Work out the finished part from the listing and answer in its coordinate system (mm). A direction names the side the tool comes from. Round coordinates to 2 decimals unless told otherwise and drop trailing zeros. Write each loop counter-clockwise with the first axis right and the second up, starting at its lowest first coordinate (ties: lowest second). Pieces come first, ordered by that corner, then holes.
1. Determine the mould class of faces 1 (the face through (-169.614, 76.799, -15.023)), 2 (the face through (-172, 11, 35.041)), 3 (the face through (-201.796, 35, 16)) for opening direction X: pulls with the +X half, pulls with the -X half, needs draft (parallel to the pull), parting line crosses it, or undercut.
2. Find section D-D (y = 57). Write down the section's boundary in (x, z), and give its area (3 significant figures).
3. Flat-ended cylindrical pins translate along their axes: pin 1 Ø4.5 at (x, z) = (-192.8, 27.04) entering from +Y; pin 2 Ø8 at (x, z) = (-194.5, 28.5) entering from +Y; pin 3 Ø5.5 at (x, z) = (-150.8, 17.04) entering from +Y; pin 4 Ø4.5 at (x, y) = (-163.5, 15) entering from +Z. Find the tip coordinate at first contact, or state that the pin passes through.
4. Straight lines are drawn through the part: probe 1 along X at (y, z) = (31.5, 13); probe 2 along X at (y, z) = (65, -5); probe 3 along Y at (x, z) = (-195.5, 28). For each, find the intervals that lie inside material, in ascending order.
5. Find section C-C (z = 23). Write down the section's boundary in (x, y).
6. Find section A-A (x = -186.5). Write down the section's boundary in (y, z).
7. A tool of negligible diameter and unlimited length cuts with its end or side. For faces 4 (the face through (-172.092, 73.446, -11.669)), 5 (the face through (-176, 11, 9.041)), 6 (the face through (-172, 12, 13)), 7 (the face through (-171.38, 32.21, 26.32)), 8 (the face through (-191.363, 10.479, 17.955)), from which of +Z, -Z, +X, -X, +Y, -Y can it reach the whole face along a straight path? Write none if from no direction.
8. Find section B-B (y = 19). Write down the section's boundary in (x, z).
```python
from build123d import *

# Parameters (mm, degrees)
SKETCH_1_W                  = 60
SKETCH_1_H                  = 26
SKETCH_1_R                  = 1.7
EXTRUDE_3_DEPTH             = 12
SKETCH_10_W                 = 5
SKETCH_10_H                 = 4
EXTRUDE_4_DEPTH             = 60
EXTRUDE_START               = -60
EXTRUDE_6_DEPTH             = 60
CUT_EXTRUDE_6_REACH         = 219.643
SKETCH_20_W                 = 5
SKETCH_20_H                 = 4
CUT_EXTRUDE_7_REACH         = 219.643
SKETCH_21_W                 = 5
SKETCH_21_H                 = 4
CUT_EXTRUDE_8_REACH         = 219.643
SKETCH_22_W                 = 5
SKETCH_22_H                 = 4
SKETCH_23_R                 = 2.25
CUT_EXTRUDE_9_DEPTH         = 10
EXTRUDE_8_REACH             = 218.77
SKETCH_24_W                 = 5
SKETCH_24_H                 = 18
EXTRUDE_8_DIRECTION_2_REACH = 218.77
EXTRUDE_START_2             = -146.796406348
EXTRUDE_9_DEPTH             = 5
SKETCH_28_W                 = 60
SKETCH_28_H                 = 9
CUT_EXTRUDE_10_DEPTH        = 26


with BuildPart() as part:
    # 草图1 → 凸台-拉伸3 (new body)
    with BuildSketch(Plane(origin=(0, 0, 0), x_dir=(1, 0, 0), z_dir=(0, 1, 0))):
        with Locations((-171.796406348, -22.041144508)):
            Rectangle(SKETCH_1_W, SKETCH_1_H)
        with Locations(Location((-150.796406348, -17.041144508, 0), (0, 0, 270))):
            Circle(SKETCH_1_R, mode=Mode.SUBTRACT)
        with Locations(Location((-150.796406348, -27.041144508, 0), (0, 0, 270))):
            Circle(SKETCH_1_R, mode=Mode.SUBTRACT)
        with Locations(Location((-192.796406348, -27.041144508, 0), (0, 0, 270))):
            Circle(SKETCH_1_R, mode=Mode.SUBTRACT)
        with Locations(Location((-198.796406348, -27.041144508, 0), (0, 0, 270))):
            Circle(SKETCH_1_R, mode=Mode.SUBTRACT)
        with Locations(Location((-198.796406348, -17.041144508, 0), (0, 0, 270))):
            Circle(SKETCH_1_R, mode=Mode.SUBTRACT)
        with Locations(Location((-192.796406348, -17.041144508, 0), (0, 0, 270))):
            Circle(SKETCH_1_R, mode=Mode.SUBTRACT)
        with Locations(Location((-144.796406348, -27.041144508, 0), (0, 0, 270))):
            Circle(SKETCH_1_R, mode=Mode.SUBTRACT)
        with Locations(Location((-144.796406348, -17.041144508, 0), (0, 0, 270))):
            Circle(SKETCH_1_R, mode=Mode.SUBTRACT)
        Polygon((-154.244576261, -28.541144508), (-153.796406348, -28.541144508), (-153.796406348, -27.585746487), (-153.796406348, -16.496542529), (-153.796406348, -15.541144508), (-154.244576261, -15.541144508), (-160.170728493, -15.541144508), (-183.422084204, -15.541144508), (-189.348236436, -15.541144508), (-189.796406348, -15.541144508), (-189.796406348, -16.496542529), (-189.796406348, -27.585746487), (-189.796406348, -28.541144508), (-189.348236436, -28.541144508), (-183.422084204, -28.541144508), (-160.170728493, -28.541144508), align=None, mode=Mode.SUBTRACT)
    extrude(amount=EXTRUDE_3_DEPTH)

    # 草图10 → 凸台-拉伸4 (add)
    with BuildSketch(Plane(origin=(0, 12, 0), x_dir=(1, 0, 0), z_dir=(0, 1, 0))):
        with Locations((-144.296406348, -11.041144508)):
            Rectangle(SKETCH_10_W, SKETCH_10_H)
        with Locations((-199.296406348, -11.041144508)):
            Rectangle(SKETCH_10_W, SKETCH_10_H)
        with Locations((-199.296406348, -33.041144508)):
            Rectangle(SKETCH_10_W, SKETCH_10_H)
        with Locations((-144.296406348, -33.041144508)):
            Rectangle(SKETCH_10_W, SKETCH_10_H)
    extrude(amount=EXTRUDE_4_DEPTH)

    # 草图16 → 凸台-拉伸6 (add)
    with BuildSketch(Plane.ZY.offset(201.796406348).offset(EXTRUDE_START)):
        Polygon((35.041144508, 23.487382081), (-19.586360532, 78.114887122), (-16.383147731, 81.318099924), (38.24435731, 26.690594883), align=None)
    extrude(amount=EXTRUDE_6_DEPTH)

    # 切除-拉伸6: up to this plane
    cut_extrude_6_end = Plane(origin=(-60.011420854, 81.318099924, -16.383147731), z_dir=(0, 0.707106781186548, 0.7071067811865472))
    # 草图20 → 切除-拉伸6 (cut, up to the surface)
    with BuildSketch(Plane(origin=(0, 72, 0), x_dir=(1, 0, 0), z_dir=(0, 1, 0)), mode=Mode.PRIVATE) as cut_extrude_6_sk1:
        with Locations((-199.296406348, -11.041144508)):
            Rectangle(SKETCH_20_W, SKETCH_20_H)
    cut_extrude_6_tool1 = split(extrude(cut_extrude_6_sk1.sketch, amount=-CUT_EXTRUDE_6_REACH, mode=Mode.PRIVATE), bisect_by=cut_extrude_6_end, keep=Keep.BOTH, mode=Mode.PRIVATE)
    add(cut_extrude_6_tool1.solids().sort_by_distance((-199.296406, 72, 11.041145))[0], mode=Mode.SUBTRACT)

    # 切除-拉伸7: up to this face of the body (flat: up to its plane)
    cut_extrude_7_end = Plane(part.part.faces().sort_by_distance((-171.967338534, 54.279900151, 10.655052042))[0])
    # 草图21 → 切除-拉伸7 (cut, up to the picked face)
    with BuildSketch(Plane(origin=(0, 72, 0), x_dir=(1, 0, 0), z_dir=(0, 1, 0)), mode=Mode.PRIVATE) as cut_extrude_7_sk1:
        with Locations((-199.296406348, -33.041144508)):
            Rectangle(SKETCH_21_W, SKETCH_21_H)
    cut_extrude_7_tool1 = split(extrude(cut_extrude_7_sk1.sketch, amount=-CUT_EXTRUDE_7_REACH, mode=Mode.PRIVATE), bisect_by=cut_extrude_7_end, keep=Keep.BOTH, mode=Mode.PRIVATE)
    add(cut_extrude_7_tool1.solids().sort_by(Axis((-199.296406, 72, 33.041145), (0, -1, 0)))[0], mode=Mode.SUBTRACT)

    # 切除-拉伸8: up to this face of the body (flat: up to its plane)
    cut_extrude_8_end = Plane(part.part.faces().sort_by_distance((-172.136158915, 54.141614108, 10.793338085))[0])
    # 草图22 → 切除-拉伸8 (cut, up to the picked face)
    with BuildSketch(Plane(origin=(0, 72, 0), x_dir=(1, 0, 0), z_dir=(0, 1, 0)), mode=Mode.PRIVATE) as cut_extrude_8_sk1:
        with Locations((-144.296406348, -11.041144508)):
            Rectangle(SKETCH_22_W, SKETCH_22_H)
    cut_extrude_8_tool1 = split(extrude(cut_extrude_8_sk1.sketch, amount=-CUT_EXTRUDE_8_REACH, mode=Mode.PRIVATE), bisect_by=cut_extrude_8_end, keep=Keep.BOTH, mode=Mode.PRIVATE)
    # 草图22 → 切除-拉伸8 (cut, up to the picked face)
    with BuildSketch(Plane(origin=(0, 72, 0), x_dir=(1, 0, 0), z_dir=(0, 1, 0)), mode=Mode.PRIVATE) as cut_extrude_8_sk2:
        with Locations((-144.296406348, -33.041144508)):
            Rectangle(SKETCH_22_W, SKETCH_22_H)
    cut_extrude_8_tool2 = split(extrude(cut_extrude_8_sk2.sketch, amount=-CUT_EXTRUDE_8_REACH, mode=Mode.PRIVATE), bisect_by=cut_extrude_8_end, keep=Keep.BOTH, mode=Mode.PRIVATE)
    add(cut_extrude_8_tool1.solids().sort_by(Axis((-144.296406, 72, 11.041145), (0, -1, 0)))[0], mode=Mode.SUBTRACT)
    add(cut_extrude_8_tool2.solids().sort_by(Axis((-144.296406, 72, 33.041145), (0, -1, 0)))[0], mode=Mode.SUBTRACT)

    # 草图23 → 切除-拉伸9 (cut)
    with BuildSketch(Plane(origin=(0, 32.467476097, 32.467476097), x_dir=(1, 0, 0), z_dir=(0, 0.7071067811865478, 0.7071067811865472))):
        Polygon((-150.696406348, 25.486333053), (-150.696406348, 4.585214747), (-192.896406348, 4.585214747), (-192.896406348, 25.486333053), (-192.896406348, 57.849143044), (-192.896406348, 60.185214747), (-150.696406348, 60.185214747), (-150.696406348, 57.849143044), align=None)
        with Locations(Location((-171.844403565, 64.635214747, 0), (0, 0, 270))):
            Circle(SKETCH_23_R)
        with Locations(Location((-171.844403565, 0.135214747, 0), (0, 0, 90))):
            Circle(SKETCH_23_R)
    extrude(amount=-CUT_EXTRUDE_9_DEPTH, mode=Mode.SUBTRACT)

    # 草图24 → 凸台-拉伸8 (add, up to next)
    with BuildSketch(Plane(origin=(0, 12, 0), x_dir=(1, 0, 0), z_dir=(0, 1, 0)), mode=Mode.PRIVATE) as extrude_8_sk1:
        with Locations((-199.296406348, -22.041144508)):
            Rectangle(SKETCH_24_W, SKETCH_24_H)
    extrude_8_tool1 = extrude(extrude_8_sk1.sketch, amount=EXTRUDE_8_REACH, mode=Mode.PRIVATE) - part.part
    add(extrude_8_tool1.solids().sort_by_distance((-199.296406, 12, 22.041145))[0])

    # 凸台-拉伸8 direction 2: up to this face of the body (flat: up to its plane)
    extrude_8_direction_2_end = Plane(part.part.faces().sort_by_distance((-142.450317657, 0, 22.041144508))[0])
    # 草图24 → 凸台-拉伸8 direction 2 (add, up to the picked face)
    with BuildSketch(Plane(origin=(0, 12, 0), x_dir=(1, 0, 0), z_dir=(0, 1, 0)), mode=Mode.PRIVATE) as extrude_8_direction_2_sk1:
        with Locations((-199.296406348, -22.041144508)):
            Rectangle(SKETCH_24_W, SKETCH_24_H)
    extrude_8_direction_2_tool1 = split(extrude(extrude_8_direction_2_sk1.sketch, amount=-EXTRUDE_8_DIRECTION_2_REACH, mode=Mode.PRIVATE), bisect_by=extrude_8_direction_2_end, keep=Keep.BOTH, mode=Mode.PRIVATE)
    add(extrude_8_direction_2_tool1.solids().sort_by(Axis((-199.296406, 12, 22.041145), (0, -1, 0)))[0])

    # 凸台-拉伸9: read off the stored shape, not the designer's step
    # 凸台-拉伸9 outline → 凸台-拉伸9 (add)
    with BuildSketch(Plane.YZ.offset(EXTRUDE_START_2)):
        Polygon((49.487382081, 9.041144508), (23.487382081, 35.041144508), (0, 35.041144508), (0, 9.041144508), align=None)
    extrude(amount=EXTRUDE_9_DEPTH)

    # 草图28 → 切除-拉伸10 (cut)
    with BuildSketch(Plane.XY.offset(35.041144508)):
        with Locations((-171.796406348, 4.5)):
            Rectangle(SKETCH_28_W, SKETCH_28_H)
    extrude(amount=-CUT_EXTRUDE_10_DEPTH, mode=Mode.SUBTRACT)


solid = part.part
```
Worked answers:
1. face 1: undercut
1. face 2: needs draft
1. face 3: pulls with the -X half
2. outline: (-201.8, 1.53) - (-192.9, 1.53) - (-192.9, 7.93) - (-201.8, 7.93) - close; (-150.7, 1.53) - (-141.8, 1.53) - (-141.8, 7.93) - (-150.7, 7.93) - close
2. area: 114 mm2
3. pin 1: stops at y = 40.14
3. pin 2: stops at y = 40.43
3. pin 3: stops at y = 50.64
3. pin 4: passes through
4. probe 1: x = -201.8 to -196.8, -146.8 to -141.8
4. probe 2: x = -201.8 to -192.9, -150.7 to -141.8
4. probe 3: y = 9 to 12, 30.53 to 36.93
5. outline: (-201.8, 9) - (-189.8, 9) - (-189.8, 12) - (-196.8, 12) - (-196.8, 35.53) - (-192.9, 35.53) - (-192.9, 41.93) - (-201.8, 41.93) - close; (-153.8, 9) - (-141.8, 9) - (-141.8, 41.93) - (-150.7, 41.93) - (-150.7, 35.53) - (-146.8, 35.53) - (-146.8, 12) - (-153.8, 12) - close
6. outline: (9, 9.04) - (12, 9.04) - (12, 15.54) - (9, 15.54) - close; (9, 28.54) - (12, 28.54) - (12, 35.04) - (9, 35.04) - close; (23.49, 35.04) - (32.51, 26.02) - (35.71, 29.23) - (26.69, 38.24) - close; (71.82, -13.29) - (78.11, -19.59) - (81.32, -16.38) - (75.02, -10.09) - close
7. face 4: +Z, -Y
7. face 5: -Z, +X, -X, -Y
7. face 6: +Z, -Z
7. face 7: -Z
7. face 8: -Y
8. outline: (-201.8, 9.04) - (-196.8, 9.04) - (-196.8, 35.04) - (-201.8, 35.04) - close; (-146.8, 9.04) - (-141.8, 9.04) - (-141.8, 35.04) - (-146.8, 35.04) - close
